Verification items for the finished model (mm, model axes). A direction names the side the tool comes from. Round coordinates to 2 decimals unless told otherwise and drop trailing zeros. Order: outer loops, then holes, each group sorted by start corner. A loop starts at its lowest first (then second) coordinate and runs counter-clockwise, first axis right, second up. Notation, with made-up numbers: (43.25, 7) -> (72.25, 7) arc R19 cw to (72.25, 18) -> close; hole circle Ø9 at (-37, 37.5). An arc over 180 degrees is marked (long way). Return JSON: item names as keys, results as strings. Group by question number.
1) Draft check along X on faces 1 (the flat face through (0, 0, 0)), 2 (the cylindrical face through (82.01, 5.37, 1.19)), 3 (the cylindrical face through (63.98, 6.21, -3.23)). Enter one of: pulls with the +X half, pulls with the -X half, needs draft (parallel to the pull), parting line crosses it, or undercut.
2) Section check B-B on x = 27. Enter the section's corners in (y, z).
3) Section check A-A on x = 55. Enter the section's corners in (y, z), plus the area to 3 significant figures.
4) Depth check by flat-ended pin: pin 1 (5 mm diameter, centred on y = -1, z = 0.5, fed in from -X); pin 2 (1.5 mm diameter, centred on x = 80.5, y = -3.5, fed in from -Z); pin 3 (1 mm diameter, centred on x = 23.5, z = 5, fed in from -Y); pin 4 (2 mm diameter, centred on x = 79.5, y = 2, fed in from -Z). Enter the tip coordinate at first touch or a pass-through.
5) Tool access check on faces 4 (the cylindrical face through (28.452, -1.322, -4.197)), 5 (the flat face through (81, -3, 5)), 6 (the cylindrical face through (88.06, 6.21, -3.23)). Record the directions out of +Z, -Z, +X, -X, +Y, -Y that give a thin tool (end or side, any length) a straight path to the whole face; none if there is none.
6) Scan lines: L1, parallel to X at y = 5.25, z = -3.75; L2, parallel to X at y = 4, z = -5.25; L3, parallel to X at y = -4, z = 3. Record each from-to range of solid material in increasing order.
```python
from build123d import *

# Parameters (mm, degrees)
FILETE1_R = 5
FILETE3_R = 1
FILETE4_R = 0.5


with BuildPart() as part:
    # Esboço1 → Revolução1 (revolve)
    with BuildSketch(Plane.XY, mode=Mode.PRIVATE) as revolu_o1_sk:
        Polygon((0, 0), (0, 1), (7.5, 1), (7.5, 3), (17.5, 4.4), (40, 4.4), (47, 7), (81, 7), (81, 5.5), (83, 5.5), (83, 7), (93, 7), (93, 0), align=None)
    revolve(revolu_o1_sk.sketch.rotate(Axis((93, 0, 0), (-1, 0, 0)), 90), axis=Axis((93, 0, 0), (-1, 0, 0)))

    # Filete1
    filete1_edges = [part.edges().sort_by_distance(p)[0] for p in [
        (40, 0, 4.4),
    ]]
    fillet(filete1_edges, radius=FILETE1_R)

    # Filete3
    filete3_edges = [part.edges().sort_by_distance(p)[0] for p in [
        (7.5, 0, 3),
    ]]
    fillet(filete3_edges, radius=FILETE3_R)

    # Filete4
    filete4_edges = [part.edges().sort_by_distance(p)[0] for p in [
        (81, 0, 7),
        (93, 0, 7),
        (83, 0, 7),
    ]]
    fillet(filete4_edges, radius=FILETE4_R)


solid = part.part
```
Check result:
{
 "1": {"face 1": "pulls with the -X half", "face 2": "undercut", "face 3": "needs draft"},
 "2": {"outline": "circle Ø8.8 at (0, 0)"},
 "3": {"outline": "circle Ø14 at (0, 0)", "area": "154 mm^2"},
 "4": {"pin 1": "x = 0", "pin 2": "z = -6.44", "pin 3": "through", "pin 4": "z = -6.93"},
 "5": {"face 4": "-X", "face 5": "none", "face 6": "+X, -X"},
 "6": {"L1": "45.52 to 81, 83 to 93", "L2": "45.92 to 80.99, 83.01 to 92.99", "L3": "41.62 to 93"}
}
